Input: part model. Units: mm. Frame: model coordinates. Face numbers are marked on the shaded views. A direction names the side the tool comes from. Give positions to 0.01 mm unless a question says otherwise; leave off trailing zeros. Loops run counter-clockwise (first coordinate to the right, second up) from the corner with the lowest first, then second, coordinate; pieces in that order, holes last. Notation, with made-up numbers: (13.5, -29) - (38.5, -29) arc R11 cw to (38.5, -24) - close; hole circle Ø7 at (49.25, 16.25). An arc over 180 degrees is marked (long way). Answer as a JSON object with one key per item and string values.
from build123d import *

# Parameters (mm, degrees)
CROQUIS1_R              = 3
SALIENTE_EXTRUIR1_DEPTH = 20
CROQUIS3_R              = 6.5
SALIENTE_EXTRUIR2_DEPTH = 12
CROQUIS4_R              = 2
SALIENTE_EXTRUIR3_DEPTH = 2.5
CROQUIS5_R              = 14.75
SALIENTE_EXTRUIR4_DEPTH = 24.5
CROQUIS6_R              = 14
SALIENTE_EXTRUIR5_DEPTH = 32.5
CROQUIS7_R              = 5.25
SALIENTE_EXTRUIR6_DEPTH = 2
CROQUIS8_R              = 1.15
SALIENTE_EXTRUIR7_DEPTH = 2
SALIENTE_EXTRUIR8_DEPTH = 2
SALIENTE_EXTRUIR9_DEPTH = 6
CORTAR_EXTRUIR1_DEPTH   = 10
CROQUIS12_W             = 0.5
CROQUIS12_H             = 0.6


with BuildPart() as part:
    # Croquis1 → Saliente-Extruir1 (new body)
    with BuildSketch(Plane.XY):
        Circle(CROQUIS1_R)
    extrude(amount=SALIENTE_EXTRUIR1_DEPTH)

    # Croquis3 → Saliente-Extruir2 (add)
    with BuildSketch(Plane.XY.offset(20)):
        Circle(CROQUIS3_R)
    extrude(amount=SALIENTE_EXTRUIR2_DEPTH)

    # Croquis4 → Saliente-Extruir3 (add)
    with BuildSketch(Plane.XY.offset(32)):
        with BuildLine():
            Line((16.5, -20), (-16.5, -20))
            ThreePointArc((-16.5, -20), (-18.974873734, -18.974873734), (-20, -16.5))
            Line((-20, -16.5), (-20, 16.5))
            ThreePointArc((-20, 16.5), (-18.974873734, 18.974873734), (-16.5, 20))
            Line((-16.5, 20), (16.5, 20))
            ThreePointArc((16.5, 20), (18.974873734, 18.974873734), (20, 16.5))
            Line((20, 16.5), (20, -16.5))
            ThreePointArc((20, -16.5), (18.974873734, -18.974873734), (16.5, -20))
        make_face()
        with Locations((15, 14.5)):
            Circle(CROQUIS4_R, mode=Mode.SUBTRACT)
        with Locations((15, -14.5)):
            Circle(CROQUIS4_R, mode=Mode.SUBTRACT)
        with Locations((-15, -14.5)):
            Circle(CROQUIS4_R, mode=Mode.SUBTRACT)
        with Locations((-15, 14.5)):
            Circle(CROQUIS4_R, mode=Mode.SUBTRACT)
    extrude(amount=SALIENTE_EXTRUIR3_DEPTH)

    # Croquis5 → Saliente-Extruir4 (add)
    with BuildSketch(Plane.XY.offset(34.5)):
        Circle(CROQUIS5_R)
    extrude(amount=SALIENTE_EXTRUIR4_DEPTH)

    # Croquis6 → Saliente-Extruir5 (add)
    with BuildSketch(Plane.XY.offset(59)):
        Circle(CROQUIS6_R)
    extrude(amount=SALIENTE_EXTRUIR5_DEPTH)

    # Croquis7 → Saliente-Extruir6 (add)
    with BuildSketch(Plane.XY.offset(91.5)):
        Circle(CROQUIS7_R)
    extrude(amount=SALIENTE_EXTRUIR6_DEPTH)

    # Croquis8 → Saliente-Extruir7 (add)
    with BuildSketch(Plane.XY.offset(93.5)):
        Circle(CROQUIS8_R)
    extrude(amount=SALIENTE_EXTRUIR7_DEPTH)

    # Croquis9 → Saliente-Extruir8 (add)
    with BuildSketch(Plane.XY.offset(91.5)):
        Polygon((8.088619231, 7.81899859), (6.351063988, 9.61646953), (7.789040741, 11.006513723), (9.526595983, 9.209042783), (11.264151225, 7.411571843), (9.826174473, 6.021527649), align=None)
        Polygon((-9.395717522, -6.673304447), (-10.736232323, -8.15756186), (-8.880910557, -9.833205361), (-7.025588791, -11.508848863), (-5.68507399, -10.02459145), (-7.540395756, -8.348947948), align=None)
    extrude(amount=SALIENTE_EXTRUIR8_DEPTH)

    # Croquis10 → Saliente-Extruir9 (add)
    with BuildSketch(Plane.XY.offset(93.5)):
        Polygon((-6.18776704, -10.581187979), (-9.898410573, -7.229900977), (-10.233539273, -7.60096533), (-6.52289574, -10.952252333), align=None)
        Polygon((6.89030527, 10.137736102), (7.249799458, 10.485247151), (10.724909943, 6.89030527), (10.365415755, 6.542794222), align=None)
    extrude(amount=SALIENTE_EXTRUIR9_DEPTH)

    # Croquis11 → Cortar-Extruir1 (cut)
    with BuildSketch(Plane(origin=(0, 0, 0), x_dir=(-1, 0, 0), z_dir=(0, 0, -1))):
        with BuildLine():
            Line((-2.598076211, 1.5), (2.598076211, 1.5))
            ThreePointArc((2.598076211, 1.5), (0, 3), (-2.598076211, 1.5))
        make_face()
    extrude(amount=-CORTAR_EXTRUIR1_DEPTH, mode=Mode.SUBTRACT)

    # Croquis12 → Cortar-Revolución1 (revolve, cut)
    with BuildSketch(Plane(origin=(0, 0, 0), x_dir=(1, 0, 0), z_dir=(0, 1, 0))):
        with Locations((-2.75, -1.7)):
            Rectangle(CROQUIS12_W, CROQUIS12_H)
    revolve(axis=Axis((0, 0, 20), (0, 0, -1)), mode=Mode.SUBTRACT)


solid = part.part
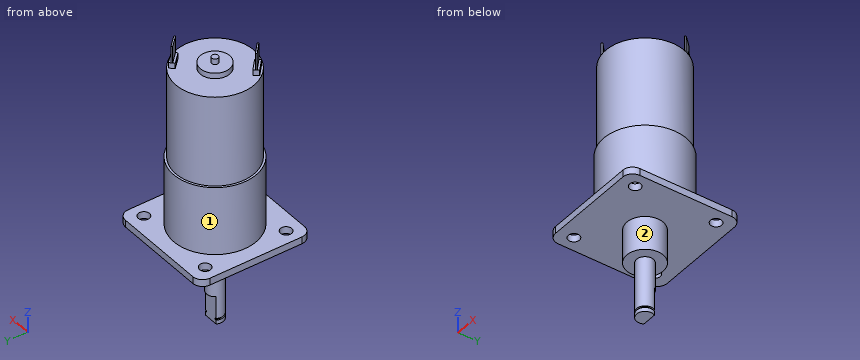
Item 1: Access query for the marked faces 1 and 2. Directions: +Z, -Z, +X, -X, +Y, -Y. A direction counts if a zero-diameter tool reaches every point of the face in a straight line with its end or side. Return the directions, or none.
Geometry check:
{"face 1": "+Z", "face 2": "-Z"}
Item 2: Cut plane C-C (z = 27). Return loops of the section in (x, y), then the cut area to 3 significant figures.
Geometry check:
{"outline": "circle Ø13 at (0, 0)", "area": "133 mm2"}
Item 3: Material intervals for line 1 (Y direction, x = -15, z = 33.65); line 2 (X direction, y = 14, z = 33); line 3 (Z direction, x = 10, y = 11), sorted ascending. Write a range as [from, to].
Geometry check:
{"line 1": "y = [-20, -16.5], [-12.5, 12.5], [16.5, 20]", "line 2": "x = [-20, -16.94], [-13.06, 13.06], [16.94, 20]", "line 3": "z = [32, 34.5]"}
Item 4: Cut plane B-B (z = 83.5). Return loops of the section in (x, y), then the cut area to 3 significant figures.
Geometry check:
{"outline": "circle Ø28 at (0, 0)", "area": "616 mm2"}
Item 5: Contact query for flat-ended pins moving along their axis: P1, Ø1.4, axis at x = -1, y = 0, coming from the +Z side; P2, Ø5, axis at y = -3.5, z = 52.5, coming from the -X side; P3, Ø6.5, axis at x = 1, y = 2.5, coming from the -Z side; P4, Ø5, axis at x = 9, y = 12.5, coming from the -Z side. Output: stop coordinate, or through.
Geometry check:
{"P1": "stops at z = 95.5", "P2": "stops at x = -14.72", "P3": "stops at z = 0", "P4": "stops at z = 32"}
